Source: CAD feature listing. Evaluate the final solid. Frame: model axes, mm. Face numbers are marked on the shaded views. Round coordinates to 2 decimals unless told otherwise and drop trailing zeros. Order: outer loops, then holes, each group sorted by start corner. A loop starts at its lowest first (then second) coordinate and runs counter-clockwise, first axis right, second up. Notation, with made-up numbers: (29.5, 1.5) - (80.5, 1.5) arc R12 ccw to (80.5, 17.5) - close; hole circle Ø8 at (-31, 58). An arc over 180 degrees is marked (long way). Return JSON: item names as keys, results as strings. Group by question number.
1) Section A-A, the plane x = 18. Return loops of the section in (y, z), plus the area to 3 significant figures.
2) Ray query, line 1 (Y direction, x = 16.25, z = 1.75); line 2 (Y direction, x = 15.75, z = 1.1); line 3 (X direction, y = 17, z = 1.9). Return the intervals inside material, ascending. Write a range as from..to.
3) Section D-D, the plane y = -3.5. Return loops of the section in (x, z).
4) Section B-B, the plane y = -14. Return loops of the section in (x, z), plus the area to 3 significant figures.
5) Section C-C, the plane z = 1.05. Return loops of the section in (x, y).
6) Mould query, pull axis X, two halves, no side actions, for the marked faces 1, 2 and 3. Classes: pulls with the +X half, pulls with the -X half, needs draft (parallel to the pull), parting line crosses it, or undercut.
7) Contact query for flat-ended pins moving along their axis: P1, Ø1.5, axis at y = -1, z = 1.5, coming from the -X side; P2, Ø1.5, axis at x = 25.5, z = 1, coming from the -Y side. Output: stop coordinate, or through.
```python
from build123d import *

# Parameters (mm, degrees)
SKETCH2_R           = 2
BOSS_EXTRUDE1_DEPTH = 2.5


with BuildPart() as part:
    # Sketch2 → Boss-Extrude1 (new body)
    with BuildSketch(Plane.XY):
        with BuildLine():
            Line((17.177810632, 20.25), (12.833062768, 20.25))
            ThreePointArc((12.833062768, 20.25), (10.711742424, 19.371320344), (9.833062768, 17.25))
            Line((9.833062768, 17.25), (9.833062768, 15.670382146))
            ThreePointArc((9.833062768, 15.670382146), (18.5, 0), (9.833062768, -15.670382146))
            Line((9.833062768, -15.670382146), (9.833062768, -17.25))
            ThreePointArc((9.833062768, -17.25), (10.711742424, -19.371320344), (12.833062768, -20.25))
            Line((12.833062768, -20.25), (17.177810632, -20.25))
            ThreePointArc((17.177810632, -20.25), (19.992731544, -19.608858273), (22.252340685, -17.811913926))
            ThreePointArc((22.252340685, -17.811913926), (28.503174274, 0), (22.252340685, 17.811913926))
            ThreePointArc((22.252340685, 17.811913926), (19.992731544, 19.608858273), (17.177810632, 20.25))
        make_face()
        with Locations((17.177810632, -15.391359244)):
            Circle(SKETCH2_R, mode=Mode.SUBTRACT)
        with Locations((17.177810632, 15.391359244)):
            Circle(SKETCH2_R, mode=Mode.SUBTRACT)
    extrude(amount=BOSS_EXTRUDE1_DEPTH)


solid = part.part
```
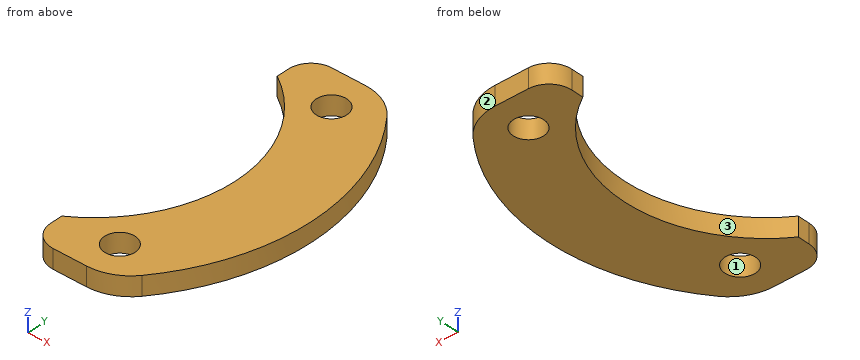
Geometry check:
{
 "1": {"outline": "(-20.2, 0) - (-17.21, 0) - (-17.21, 2.5) - (-20.2, 2.5) - close; (-13.57, 0) - (-4.27, 0) - (-4.27, 2.5) - (-13.57, 2.5) - close; (4.27, 0) - (13.57, 0) - (13.57, 2.5) - (4.27, 2.5) - close; (17.21, 0) - (20.2, 0) - (20.2, 2.5) - (17.21, 2.5) - close", "area": "61.4 mm2"},
 "2": {"line 1": "-20.25..-17.16, -13.62..-8.84, 8.84..13.62, 17.16..20.25", "line 2": "-20.25..-16.79, -13.99..-9.71, 9.71..13.99, 16.79..20.25", "line 3": "9.83..15.99, 18.37..22.88"},
 "3": {"outline": "(18.17, 0) - (28.29, 0) - (28.29, 2.5) - (18.17, 2.5) - close"},
 "4": {"outline": "(12.09, 0) - (15.74, 0) - (15.74, 2.5) - (12.09, 2.5) - close; (18.61, 0) - (24.83, 0) - (24.83, 2.5) - (18.61, 2.5) - close", "area": "24.7 mm2"},
 "5": {"outline": "(9.83, -17.25) arc R3 ccw to (12.83, -20.25) - (17.18, -20.25) arc R6.5 ccw to (22.25, -17.81) arc R28.5 ccw to (22.25, 17.81) arc R6.5 ccw to (17.18, 20.25) - (12.83, 20.25) arc R3 ccw to (9.83, 17.25) - (9.83, 15.67) arc R18.5 cw to (9.83, -15.67) - close; hole circle Ø4 at (17.18, -15.39); hole circle Ø4 at (17.18, 15.39)"},
 "6": {"face 1": "undercut", "face 2": "pulls with the +X half", "face 3": "pulls with the -X half"},
 "7": {"P1": "x = 18.42", "P2": "y = -14.14"}
}
